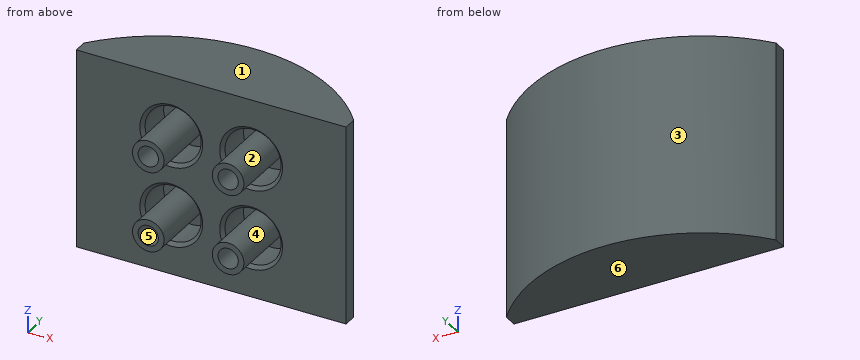
```python
from build123d import *

# Parameters (mm, degrees)
SKETCH1_W           = 59.7
SKETCH1_H           = 3
BOSS_EXTRUDE1_DEPTH = 44
SKETCH2_R           = 3.5
SKETCH2_R_2         = 2.25
BOSS_EXTRUDE2_DEPTH = 9
CUT_EXTRUDE1_START  = -8
SKETCH3_R           = 6.2
SKETCH3_R_2         = 3.5
CUT_EXTRUDE1_DEPTH  = 8
CHAMFER1_SIZE       = 0.75


with BuildPart() as part:
    # Sketch1 → Boss-Extrude1 (new body)
    with BuildSketch(Plane.XY):
        with BuildLine():
            ThreePointArc((29.85, 3), (0, 17.273040059), (-29.85, 3))
            Line((-29.85, 3), (29.85, 3))
        make_face()
        with Locations((0, 1.5)):
            Rectangle(SKETCH1_W, SKETCH1_H)
    extrude(amount=BOSS_EXTRUDE1_DEPTH)

    # Sketch2 → Boss-Extrude2 (add)
    # profile 1 of 4: a face of its own
    with BuildSketch(Plane.XZ):
        with Locations(Location((8.838834765, 30.838834765, 0), (0, 0, 180))):
            Circle(SKETCH2_R)
        with Locations((8.838834765, 30.838834765)):
            Circle(SKETCH2_R_2, mode=Mode.SUBTRACT)
    # profile 2 of 4: a face of its own
    with BuildSketch(Plane.XZ):
        with Locations(Location((8.838834765, 13.161165235, 0), (0, 0, 180))):
            Circle(SKETCH2_R)
        with Locations((8.838834765, 13.161165235)):
            Circle(SKETCH2_R_2, mode=Mode.SUBTRACT)
    # profile 3 of 4: a face of its own
    with BuildSketch(Plane.XZ):
        with Locations(Location((-8.838834765, 13.161165235, 0), (0, 0, 180))):
            Circle(SKETCH2_R)
        with Locations((-8.838834765, 13.161165235)):
            Circle(SKETCH2_R_2, mode=Mode.SUBTRACT)
    # profile 4 of 4: a face of its own
    with BuildSketch(Plane.XZ):
        with Locations(Location((-8.838834765, 30.838834765, 0), (0, 0, 180))):
            Circle(SKETCH2_R)
        with Locations((-8.838834765, 30.838834765)):
            Circle(SKETCH2_R_2, mode=Mode.SUBTRACT)
    extrude(amount=BOSS_EXTRUDE2_DEPTH)

    # Sketch3 → Cut-Extrude1 (cut)
    # profile 1 of 4: a face of its own
    with BuildSketch(Plane.XZ.offset(CUT_EXTRUDE1_START)):
        with Locations((-8.838834765, 30.838834765)):
            Circle(SKETCH3_R)
        with Locations((-8.838834765, 30.838834765)):
            Circle(SKETCH3_R_2, mode=Mode.SUBTRACT)
    # profile 2 of 4: a face of its own
    with BuildSketch(Plane.XZ.offset(CUT_EXTRUDE1_START)):
        with Locations((8.838834765, 30.838834765)):
            Circle(SKETCH3_R)
        with Locations((8.838834765, 30.838834765)):
            Circle(SKETCH3_R_2, mode=Mode.SUBTRACT)
    # profile 3 of 4: a face of its own
    with BuildSketch(Plane.XZ.offset(CUT_EXTRUDE1_START)):
        with Locations((8.838834765, 13.161165235)):
            Circle(SKETCH3_R)
        with Locations((8.838834765, 13.161165235)):
            Circle(SKETCH3_R_2, mode=Mode.SUBTRACT)
    # profile 4 of 4: a face of its own
    with BuildSketch(Plane.XZ.offset(CUT_EXTRUDE1_START)):
        with Locations((-8.838834765, 13.161165235)):
            Circle(SKETCH3_R)
        with Locations((-8.838834765, 13.161165235)):
            Circle(SKETCH3_R_2, mode=Mode.SUBTRACT)
    extrude(amount=CUT_EXTRUDE1_DEPTH, mode=Mode.SUBTRACT)

    # Chamfer1
    chamfer1_edges = [part.edges().sort_by_distance(p)[0] for p in [
        (-15.038834765, 0, 13.161165235),
        (2.638834765, 0, 13.161165235),
        (2.638834765, 0, 30.838834765),
        (-15.038834765, 0, 30.838834765),
    ]]
    chamfer(chamfer1_edges, length=CHAMFER1_SIZE)


solid = part.part
```
The model under review builds one solid part; all positions refer to its coordinate system, in mm. Face numbers are marked on the shaded views. A direction names the side the tool comes from. Round coordinates to 2 decimals unless told otherwise and drop trailing zeros. Loops run counter-clockwise (first coordinate to the right, second up) from the corner with the lowest first, then second, coordinate; pieces in that order, holes last. Notation, with made-up numbers: M 89.25,-13.75 L 107.25,-13.75 A23 cw 107.25,18.25 Z; hole C 39,40 d2. An arc over 180 degrees is marked long. Put each result on its own line as item: value.
Q1. To check wall thickness, follow L1, parallel to Z at x = 13, y = 7 (3 decimals); L2, parallel to X at y = -3.5, z = 15; L3, parallel to X at y = -7.25, z = 31.5. State the ranges of each line that lie inside material, in increasing order.
Result set:
L1: z = 0 to 8.565, 17.757 to 26.243, 35.435 to 44
L2: x = -11.82 to -10.14, -7.54 to -5.86, 5.86 to 7.54, 10.14 to 11.82
L3: x = -12.28 to -10.99, -6.69 to -5.4, 5.4 to 6.69, 10.99 to 12.28
Q2. For pin 1 (10 mm diameter, centred on y = 13, z = 37.5, fed in from -X); pin 2 (10 mm diameter, centred on x = 16, z = 10, fed in from +Y); pin 3 (2 mm diameter, centred on x = -8, z = 31.5, fed in from -Y); pin 4 (22 mm diameter, centred on x = -8, z = 19, fed in from -Y), all flat-tipped, find the tip position at first contact; note any pin that passes through.
Result set:
pin 1: stops at x = -25.01
pin 2: stops at y = 15.66
pin 3: stops at y = 0
pin 4: stops at y = -9
Q3. Consider section D-D, the plane x = 21. Give the boundary of the cut face in (y, z), then the cut area to 3 significant figures.
Result set:
outline: M 0,0 L 11.01,0 L 11.01,44 L 0,44 Z
area: 485 mm²
Q4. Mouldability with a two-part tool opening along X and no side actions: class the marked faces 3, 4, 5 and 6 as released by +X, released by -X, zero draft, split by the parting line, or undercut.
Result set:
face 3: split by the parting line
face 4: undercut
face 5: undercut
face 6: zero draft
Q5. Consider section B-B, the plane z = 4. Give the boundary of the cut face in (x, y), then the cut area to 3 significant figures.
Result set:
outline: M -29.85,0 L 29.85,0 L 29.85,3 A38.35 ccw -29.85,3 Z
area: 772 mm²
Q6. Machinability: for the marked faces 1 and 2, which of the approach directions +Z, -Z, +X, -X, +Y, -Y give a long, thin tool a straight path to every point of the face, cutting with its end or side? Answer none if there is none.
Result set:
face 1: +Z, +X, -X, +Y, -Y
face 2: -Y
Q7. Consider section A-A, the plane y = 5.5. Count the separate pieces of the cut face and the enclosed holes in it, then the cut area to 3 significant figures.
Result set:
separate pieces: 5
enclosed holes: 4
area: 2,100 mm²
